Part model, mm, in its own coordinate system. A direction names the side the tool comes from. Coordinates: 2 decimals unless noted, no trailing zeros. Loops run counter-clockwise (first coordinate to the right, second up) from the corner with the lowest first, then second, coordinate; pieces in that order, holes last. Notation, with made-up numbers: (38.5, 40.5) -> (57.5, 40.5) arc R11 cw to (57.5, 55.5) -> close; hole circle Ø9 at (89.25, -38.5). An arc over 180 degrees is marked (long way). Use one line per item in the form item = value. Start each with the question number.
(1) Band-saw the part on A-A on y = 4. Give the cut face in (x, z).
(2) 3-axis set-ups, long thin cutter, end or side, ignore diameter. For faces 4 (the flat face through (0, 0, 2.5)), 5 (the flat face through (0, 0, 4.5)): which of +Z, -Z, +X, -X, +Y, -Y reach the whole face in a straight line?
(3) Drill centre lines: L1, parallel to Y at x = 0, z = 0.75; L2, parallel to Z at x = 12.5, y = -3.75; L3, parallel to X at y = -3.25, z = 3.75. Where is each one in solid material? Low to high. Write a range as [from, to].
(4) Band-saw the part on B-B on x = 0. Give the cut face in (y, z).
(5) Mould opens along Y. For faces 1 (the cylindrical face through (-0.34, -1.55, 1.23)), 2 (the flat face through (0, 2, 0)), 3 (the cylindrical face through (-14.985, 0.66, 3.486)) say: +Y half, -Y half, draft (parallel to the pull), parting line (faces both ways), or undercut.
(6) Band-saw the part on D-D on z = 3.6. Give the cut face in (x, y), then the cut area to 3 significant figures.
(7) Pin check, flat tips, straight feed: P1, Ø9, axis at x = -3.5, y = 4.5, coming from the -Z side; P2, Ø2, axis at y = -4, z = 3, coming from the -X side; P3, Ø1, axis at x = 0.5, y = -0.5, coming from the -Z side. Stop position of each tip, or through.
(8) Band-saw the part on C-C on z = 1.85. Give the cut face in (x, y) (1 decimal), then the cut area to 3 significant figures.
```python
from build123d import *

# Parameters (mm, degrees)
F0_R     = 7.5
F0_R_2   = 1.5875
F1_DEPTH = 2.5
F2_R     = 15
F2_R_2   = 7.5
F3_DEPTH = 2


with BuildPart() as f1:
    # F0 (on Top) → F1 (new body)
    with BuildSketch(Plane.XY):
        Circle(F0_R)
        Circle(F0_R_2, mode=Mode.SUBTRACT)
    extrude(amount=F1_DEPTH)

    # F2 (on face) → F3 (join)
    with BuildSketch(Plane.XY.offset(2.5)):
        Circle(F2_R)
        Circle(F2_R_2, mode=Mode.SUBTRACT)
        Circle(F2_R)
    extrude(amount=F3_DEPTH)


solid = f1.part
```
A:
q1.outline = (-14.46, 2.5) -> (-6.34, 2.5) -> (-6.34, 0) -> (6.34, 0) -> (6.34, 2.5) -> (14.46, 2.5) -> (14.46, 4.5) -> (-14.46, 4.5) -> close
q2.face_4 = -Z
q2.face_5 = +Z, +X, -X, +Y, -Y
q3.L1 = [-7.5, -1.59], [1.59, 7.5]
q3.L2 = [2.5, 4.5]
q3.L3 = [-14.64, 14.64]
q4.outline = (-15, 2.5) -> (-7.5, 2.5) -> (-7.5, 0) -> (-1.59, 0) -> (-1.59, 2.5) -> (1.59, 2.5) -> (1.59, 0) -> (7.5, 0) -> (7.5, 2.5) -> (15, 2.5) -> (15, 4.5) -> (-15, 4.5) -> close
q5.face_1 = undercut
q5.face_2 = draft
q5.face_3 = parting line
q6.outline = circle Ø30 at (0, 0)
q6.area = 707 mm²
q7.P1 = 0
q7.P2 = -14.7
q7.P3 = 2.5
q8.outline = circle Ø15 at (0, 0); hole circle Ø3.2 at (0, 0)
q8.area = 169 mm²
